```python
from build123d import *

# Parameters (mm, degrees)
SKETCH1_W           = 10
SKETCH1_H           = 120
BOSS_EXTRUDE1_DEPTH = 55
SKETCH2_W           = 42
SKETCH2_H           = 8
BOSS_EXTRUDE2_DEPTH = 42
SKETCH3_R           = 7.5
CUT_EXTRUDE1_DEPTH  = 8
SKETCH5_W           = 60
SKETCH5_H           = 145
BOSS_EXTRUDE4_DEPTH = 10
SKETCH6_R           = 2.75
CUT_EXTRUDE2_DEPTH  = 10
SKETCH7_R           = 2.5
CUT_EXTRUDE3_DEPTH  = 10


with BuildPart() as part:
    # Sketch1 → Boss-Extrude1 (new body)
    with BuildSketch(Plane.XY):
        with Locations((3, 50.202041029)):
            Rectangle(SKETCH1_W, SKETCH1_H)
    extrude(amount=BOSS_EXTRUDE1_DEPTH)

    # Sketch2 → Boss-Extrude2 (add)
    with BuildSketch(Plane(origin=(8, 0, 0), x_dir=(0, 0, -1), z_dir=(1, 0, 0))):
        with Locations((-34, 14.202041029)):
            Rectangle(SKETCH2_W, SKETCH2_H)
    extrude(amount=BOSS_EXTRUDE2_DEPTH)

    # Sketch3 → Cut-Extrude1 (cut)
    with BuildSketch(Plane.XZ.offset(-10.202041029)):
        with Locations((29, 34)):
            Circle(SKETCH3_R)
    extrude(amount=-CUT_EXTRUDE1_DEPTH, mode=Mode.SUBTRACT)

    # Sketch5 → Boss-Extrude4 (add)
    with BuildSketch(Plane.XY.offset(55)):
        with Locations((28, 62.702041029)):
            Rectangle(SKETCH5_W, SKETCH5_H)
    extrude(amount=BOSS_EXTRUDE4_DEPTH)

    # Sketch6 → Cut-Extrude2 (cut)
    with BuildSketch(Plane.XY.offset(65)):
        with Locations((27, 114.702041029)):
            Circle(SKETCH6_R)
        with Locations((27, 82.702041029)):
            Circle(SKETCH6_R)
        with Locations((27, 42.702041029)):
            Circle(SKETCH6_R)
        with Locations((27, 10.702041029)):
            Circle(SKETCH6_R)
    extrude(amount=-CUT_EXTRUDE2_DEPTH, mode=Mode.SUBTRACT)

    # Sketch7 → Cut-Extrude3 (cut)
    with BuildSketch(Plane(origin=(8, 0, 0), x_dir=(0, 0, -1), z_dir=(1, 0, 0))):
        with Locations((-47, 102.202041029)):
            Circle(SKETCH7_R)
        with Locations((-8, 102.202041029)):
            Circle(SKETCH7_R)
        with Locations((-47, -1.797958971)):
            Circle(SKETCH7_R)
        with Locations((-8, -1.797958971)):
            Circle(SKETCH7_R)
    extrude(amount=-CUT_EXTRUDE3_DEPTH, mode=Mode.SUBTRACT)


solid = part.part
```
Geometry check sheet. Reference: the model listing, model coordinates, mm. A direction names the side the tool comes from. Give positions to 0.01 mm unless a question says otherwise; leave off trailing zeros. Order: outer loops, then holes, each group sorted by start corner. A loop starts at its lowest first (then second) coordinate and runs counter-clockwise, first axis right, second up. Notation, with made-up numbers: (5.25, -20) -> (45.25, -20) arc R18 cw to (45.25, -11) -> close; hole circle Ø4 at (5.5, 77.5). An arc over 180 degrees is marked (long way). Write each question's results on one line, items separated by ' | '. Start each with the question number.
(1) Sectioned sample at C-C (x = 19). Enter the section's corners in (y, z), plus the area to 3 significant figures.
(2) Sectioned sample at D-D (z = 34). Enter the section's corners in (x, y).
(3) Sectioned sample at A-A (z = 8). Enter the section's corners in (x, y), plus the area to 3 significant figures.
(4) Gauge pin test, flat ends, axial feed: P1, Ø6, axis at y = -1.8, z = 8, coming from the -X side; P2, Ø2.5, axis at x = 28, y = 16, coming from the -Z side; P3, Ø6, axis at x = 31.5, z = 10.5, coming from the -Y side; P4, Ø2, axis at x = 49.5, y = 94, coming from the -Z side. Record the tip position at first contact, or that the pin passes through.
(5) Scan lines: line 1 (Y direction, x = 27, z = 62); line 2 (Y direction, x = 2.25, z = 8); line 3 (Z direction, x = 29, y = 15). Record each from-to range of solid material in increasing order.
(6) Sectioned sample at B-B (y = 15.5). Enter the section's corners in (x, z).
(7) Mould release check, pull along Y, two halves, no side actions. Record for faces 6 (the face through (3, 110.202, 27)), 7 (the face through (27, 11, 55)), 8 (the face through (27.37, 14.15, 26.68)), 9 (the face through (3.07, -2.755, 44.691)): pulls with the +Y half, pulls with the -Y half, needs draft (parallel to the pull), parting line crosses it, or undercut.
(8) Access from +Z, -Z, +X, -X, +Y, -Y to the whole of each face (thin tool, end or side, straight path). Record for faces 1 (the face through (19, 10.202, 34)), 2 (the face through (29, 14, 13)), 3 (the face through (28, 135.202, 60)), 4 (the face through (24.253, 10.823, 60.07)), 5 (the face through (19, 18.202, 34)).
Answer below:
1) outline: (-9.8, 55) -> (10.2, 55) -> (10.2, 13) -> (18.2, 13) -> (18.2, 55) -> (135.2, 55) -> (135.2, 65) -> (-9.8, 65) -> close | area: 1,790 mm2
2) outline: (-2, -9.8) -> (8, -9.8) -> (8, 10.2) -> (21.5, 10.2) -> (21.5, 18.2) -> (8, 18.2) -> (8, 110.2) -> (-2, 110.2) -> close; (36.5, 10.2) -> (50, 10.2) -> (50, 18.2) -> (36.5, 18.2) -> close
3) outline: (-2, -9.8) -> (8, -9.8) -> (8, -4.3) -> (-2, -4.3) -> close; (-2, 0.7) -> (8, 0.7) -> (8, 99.7) -> (-2, 99.7) -> close; (-2, 104.7) -> (8, 104.7) -> (8, 110.2) -> (-2, 110.2) -> close | area: 1,100 mm2
4) P1: x = -2 | P2: z = 13 | P3: y = 10.2 | P4: z = 55
5) line 1: -9.8 to 7.95, 13.45 to 39.95, 45.45 to 79.95, 85.45 to 111.95, 117.45 to 135.2 | line 2: -9.8 to -4.3, 0.7 to 99.7, 104.7 to 110.2 | line 3: 13 to 26.5, 41.5 to 65
6) outline: (-2, 0) -> (8, 0) -> (8, 13) -> (50, 13) -> (50, 55) -> (58, 55) -> (58, 65) -> (-2, 65) -> close; hole circle Ø15 at (29, 34)
7) face 6: pulls with the +Y half | face 7: undercut | face 8: needs draft | face 9: undercut
8) face 1: -Z, +X, -Y | face 2: -Z, +X, +Y, -Y | face 3: +Z, -Z, +X, -X, +Y | face 4: +Z | face 5: -Z, +X, +Y
